```python
from build123d import *

# Parameters (mm, degrees)
SKETCH_1_W          = 40
SKETCH_1_H          = 39
SKETCH_1_R          = 2
EXTRUDE_1_DEPTH     = 8
SKETCH_2_R          = 1.75
CUT_EXTRUDE_1_DEPTH = 8
CUT_EXTRUDE_START   = -31
SKETCH_2_3_R        = 1.75
CUT_EXTRUDE_2_DEPTH = 8
SKETCH_4_R          = 10
CUT_EXTRUDE_3_DEPTH = 10
CUT_EXTRUDE_5_DEPTH = 10


with BuildPart() as part:
    # 草图1 → 凸台-拉伸1 (new body)
    with BuildSketch(Plane(origin=(0, 0, 0), x_dir=(1, 0, 0), z_dir=(0, 1, 0))):
        with Locations((-2, 4)):
            Rectangle(SKETCH_1_W, SKETCH_1_H)
        with Locations(Location((0, 0, 0), (0, 0, 270))):
            Circle(SKETCH_1_R, mode=Mode.SUBTRACT)
    extrude(amount=EXTRUDE_1_DEPTH)

    # 草图2 → 切除-拉伸1 (cut)
    with BuildSketch(Plane.XY.offset(15.5)):
        with Locations((9, 4)):
            Circle(SKETCH_2_R)
        with Locations((-16, 4)):
            Circle(SKETCH_2_R)
    extrude(amount=-CUT_EXTRUDE_1_DEPTH, mode=Mode.SUBTRACT)

    # 草图2<3> → 切除-拉伸2 (cut)
    with BuildSketch(Plane.XY.offset(15.5).offset(CUT_EXTRUDE_START)):
        with Locations((9, 4)):
            Circle(SKETCH_2_3_R)
        with Locations((-16, 4)):
            Circle(SKETCH_2_3_R)
    extrude(amount=-CUT_EXTRUDE_2_DEPTH, mode=Mode.SUBTRACT)

    # 草图4 → 切除-拉伸3 (cut)
    with BuildSketch(Plane(origin=(0, 0, 0), x_dir=(-1, 0, 0), z_dir=(0, -1, 0))):
        with Locations((22, 4)):
            Circle(SKETCH_4_R)
    extrude(amount=-CUT_EXTRUDE_3_DEPTH, mode=Mode.SUBTRACT)

    # 草图6 → 切除-拉伸5 (cut)
    with BuildSketch(Plane(origin=(0, 8, 0), x_dir=(1, 0, 0), z_dir=(0, 1, 0))):
        with BuildLine():
            Line((13, -5.5), (13, 13.5))
            ThreePointArc((13, 13.5), (18, 18.5), (23, 13.5))
            Line((23, 13.5), (23, -5.5))
            ThreePointArc((23, -5.5), (18, -10.5), (13, -5.5))
        make_face()
    extrude(amount=-CUT_EXTRUDE_5_DEPTH, mode=Mode.SUBTRACT)


solid = part.part
```
Can you work these out from the model? Positions are in its coordinate system, mm. A direction names the side the tool comes from. Coordinates: 2 decimals unless noted, no trailing zeros. Loops run counter-clockwise (first coordinate to the right, second up) from the corner with the lowest first, then second, coordinate; pieces in that order, holes last. Notation, with made-up numbers: (15.25, 53.25) - (36.25, 53.25) arc R12 ccw to (36.25, 61.25) - close; hole circle Ø9 at (-40, 31). An arc over 180 degrees is marked (long way). Use a Markdown table: item, result.
Item 1: I want a section at A-A on x = 0. Please give me the cut outline in (y, z).
Numbers:
| item | result |
|---|---|
| outline | (0, -23.5) - (8, -23.5) - (8, -2) - (0, -2) - close; (0, 2) - (8, 2) - (8, 15.5) - (0, 15.5) - close |
Item 2: We'd pull the mould along Y, two halves only. Please class faces 1 (the face through (-2, 4, 0)), 2 (the face through (-2, 0, -4)), 3 (the face through (9, 4, -15.5)): released by +Y, released by -Y, zero draft, split by the parting line, or undercut.
Numbers:
| item | result |
|---|---|
| face 1 | zero draft |
| face 2 | released by -Y |
| face 3 | undercut |
Item 3: I want a section at C-C on z = 0. Please give me the cut outline in (x, y).
Numbers:
| item | result |
|---|---|
| outline | (-12.83, 0) - (-2, 0) - (-2, 8) - (-12.83, 8) - close; (2, 0) - (13, 0) - (13, 8) - (2, 8) - close |
Item 4: I want a section at D-D on x = 9. Please give me the cut outline in (y, z).
Numbers:
| item | result |
|---|---|
| outline | (0, -23.5) - (2.25, -23.5) - (2.25, -15.5) - (5.75, -15.5) - (5.75, -23.5) - (8, -23.5) - (8, 15.5) - (5.75, 15.5) - (5.75, 7.5) - (2.25, 7.5) - (2.25, 15.5) - (0, 15.5) - close |
Item 5: Will these pins go through, and if not, where does the flat tip stop? pin 1 (2 mm diameter, centred on y = 4, z = 4.5, fed in from +X); pin 2 (2 mm diameter, centred on x = -16, y = 4, fed in from +Z); pin 3 (1 mm diameter, centred on x = 9.5, y = 4, fed in from -Z).
Numbers:
| item | result |
|---|---|
| pin 1 | stops at x = 13 |
| pin 2 | stops at z = 7.5 |
| pin 3 | stops at z = -15.5 |
Item 6: For faces 4 (the face through (9.81, 2.45, -19.44)), 5 (the face through (13, 4, -4)), 6 (the face through (-22, 4, -19)), 7 (the face through (9, 4, 7.5)), which set-ups out of +Z, -Z, +X, -X, +Y, -Y let a thin tool reach every point of the face, with its end or its side?
Numbers:
| item | result |
|---|---|
| face 4 | -Z |
| face 5 | +X, +Y, -Y |
| face 6 | +Z, -Z, -X, +Y, -Y |
| face 7 | +Z |
Item 7: I want a section at B-B on y = 7.25. Please give me the cut outline in (x, z), and give its area (3 significant figures).
Numbers:
| item | result |
|---|---|
| outline | (-22, -23.5) - (18, -23.5) - (18, -18.5) arc R5 cw to (13, -13.5) - (13, 5.5) arc R5 cw to (18, 10.5) - (18, 15.5) - (-22, 15.5) - (-22, 6) arc R10 cw to (-22, -14) - close; hole circle Ø4 at (0, 0) |
| area | 1,260 mm2 |
Item 8: If I drill on probe 1 along Y at (x, z) = (9, 13); probe 2 along X at (y, z) = (4.5, 14); probe 3 along X at (y, z) = (3, 12.5), over which ranges is the centre line in solid material (lowest first)? Write a range as from..to.
Numbers:
| item | result |
|---|---|
| probe 1 | y = 0..2.25, 5.75..8 |
| probe 2 | x = -22..-17.68, -14.32..7.32, 10.68..18 |
| probe 3 | x = -22..-17.44, -14.56..7.56, 10.44..18 |
